For this review, take the finished solid that the model builds, in its own axes (mm). Face numbers are marked on the shaded views. A direction names the side the tool comes from. Coordinates: 2 decimals unless noted, no trailing zeros. Write each loop counter-clockwise with the first axis right and the second up, starting at its lowest first coordinate (ties: lowest second). Pieces come first, ordered by that corner, then holes. Notation, with made-up numbers: (19.25, 41) - (29.25, 41) arc R13 cw to (29.25, 56) - close; hole circle Ø9 at (5, 26.5). An arc over 180 degrees is marked (long way). Write each question's results on one line, items separated by ' | '.
from build123d import *

# Parameters (mm, degrees)
SKETCH1_W           = 13.2
SKETCH1_H           = 9.1
BOSS_EXTRUDE1_DEPTH = 1
SKETCH2_W           = 3.5
SKETCH2_H           = 4.2
BOSS_EXTRUDE2_DEPTH = 1.65
SKETCH3_W           = 0.6
SKETCH3_H           = 1.2
BOSS_EXTRUDE3_DEPTH = 0.6
SKETCH4_W           = 4.618980196
SKETCH4_H           = 7.488452384
BOSS_EXTRUDE4_DEPTH = 0.35
SKETCH5_W           = 0.529853481
SKETCH5_H           = 0.437759734
SKETCH5_H_2         = 0.437759735
BOSS_EXTRUDE5_DEPTH = 1.35


with BuildPart() as part:
    # Sketch1 → Boss-Extrude1 (new body)
    with BuildSketch(Plane(origin=(0, 0, 0), x_dir=(1, 0, 0), z_dir=(0, 1, 0))):
        Rectangle(SKETCH1_W, SKETCH1_H)
    extrude(amount=BOSS_EXTRUDE1_DEPTH)

    # Sketch2 → Boss-Extrude2 (add)
    with BuildSketch(Plane(origin=(0, 1, 0), x_dir=(1, 0, 0), z_dir=(0, 1, 0))):
        Rectangle(SKETCH2_W, SKETCH2_H)
    extrude(amount=BOSS_EXTRUDE2_DEPTH)

    # Sketch3 → Boss-Extrude3 (add)
    with BuildSketch(Plane(origin=(0, 1, 0), x_dir=(1, 0, 0), z_dir=(0, 1, 0))):
        with Locations((5.310699057, 0)):
            Rectangle(SKETCH3_W, SKETCH3_H)
    extrude(amount=BOSS_EXTRUDE3_DEPTH)

    # Sketch4 → Boss-Extrude4 (add)
    with BuildSketch(Plane.XZ):
        with Locations((0, 4.449008393)):
            Rectangle(SKETCH4_W, SKETCH4_H)
    extrude(amount=BOSS_EXTRUDE4_DEPTH)

    # Sketch5 → Boss-Extrude5 (add)
    with BuildSketch(Plane(origin=(0, 0, 0), x_dir=(1, 0, 0), z_dir=(0, 1, 0))):
        with Locations((-2.01492674, 1.370758696)):
            Rectangle(SKETCH5_W, SKETCH5_H)
        with Locations((-2.01492674, 0.456919566)):
            Rectangle(SKETCH5_W, SKETCH5_H_2)
        with Locations((2.01492674, 0.456919566)):
            Rectangle(SKETCH5_W, SKETCH5_H_2)
        with Locations((2.01492674, 1.370758696)):
            Rectangle(SKETCH5_W, SKETCH5_H)
        with Locations((2.01492674, -1.370758696)):
            Rectangle(SKETCH5_W, SKETCH5_H)
        with Locations((2.01492674, -0.456919566)):
            Rectangle(SKETCH5_W, SKETCH5_H_2)
        with Locations((-2.01492674, -0.456919566)):
            Rectangle(SKETCH5_W, SKETCH5_H_2)
        with Locations((-2.01492674, -1.370758696)):
            Rectangle(SKETCH5_W, SKETCH5_H)
    extrude(amount=BOSS_EXTRUDE5_DEPTH)


solid = part.part
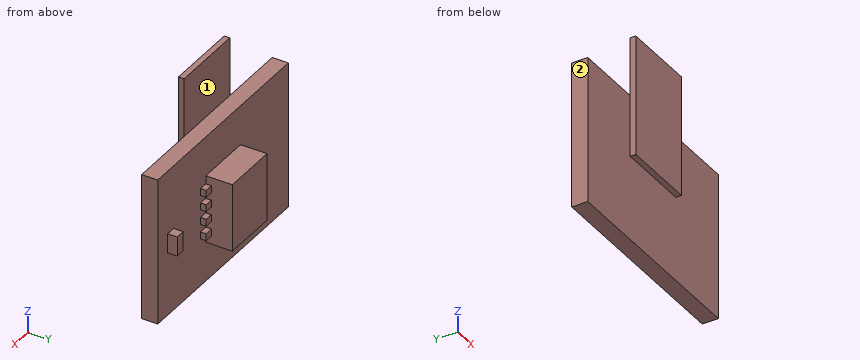
Q1. Wall thickness on line 1 along Z through (x, y) = (5.75, 0.7); line 2 along X through (y, z) = (1.55, 0.5); line 3 along Y through (x, z) = (-1.5, 5.5): over which ranges is each line inside the solid? List them lowest first. Write a range as from..to.
Results found:
line 1: -4.55..4.55 | line 2: -1.75..1.75, 5.01..5.61 | line 3: -0.35..0
Q2. For pin 1 (3 mm diameter, centred on x = 3, z = 3.5, fed in from -Y); pin 2 (0.7 mm diameter, centred on x = 5, z = 0.5, fed in from +Y); pin 3 (1.5 mm diameter, centred on x = 4, z = 1.5, fed in from -Y), all flat-tipped, find the tip position at first contact; note any pin that passes through.
Results found:
pin 1: y = -0.35 | pin 2: y = 1.6 | pin 3: y = 0
Q3. For the marked faces 1 and 2, list the 3-axis set-ups (+Z, -Z, +X, -X, +Y, -Y) from which the entire face can be reached by the end or side of a thin tool; tool diameter is ignored.
Results found:
face 1: +Z, +X, -X, +Y | face 2: +Z, -Z, -X, +Y, -Y
Q4. Take a section at B-B on x = -1.5. State the section outline as (y, z) points.
Results found:
outline: (-0.35, 0.7) - (0, 0.7) - (0, -4.55) - (1, -4.55) - (1, -2.1) - (2.65, -2.1) - (2.65, 2.1) - (1, 2.1) - (1, 4.55) - (0, 4.55) - (0, 8.19) - (-0.35, 8.19) - close
Q5. Take a section at D-D on z = -1. State the section outline as (x, y) points, plus the area to 3 significant figures.
Results found:
outline: (-6.6, 0) - (6.6, 0) - (6.6, 1) - (1.75, 1) - (1.75, 2.65) - (-1.75, 2.65) - (-1.75, 1) - (-6.6, 1) - close | area: 19.0 mm2
Q6. Take a section at C-C on y = 2.45. State the section outline as (x, z) points, plus the area to 3 significant figures.
Results found:
outline: (-1.75, -2.1) - (1.75, -2.1) - (1.75, 2.1) - (-1.75, 2.1) - close | area: 14.7 mm2
Q7. Take a section at A-A on z = 1.75. State the section outline as (x, y) points.
Results found:
outline: (-6.6, 0) - (-2.31, 0) - (-2.31, -0.35) - (2.31, -0.35) - (2.31, 0) - (6.6, 0) - (6.6, 1) - (1.75, 1) - (1.75, 2.65) - (-1.75, 2.65) - (-1.75, 1) - (-6.6, 1) - close
